Input: part model. Units: mm. Frame: model coordinates. A direction names the side the tool comes from. Give positions to 0.01 mm unless a question says otherwise; leave off trailing zeros. Loops run counter-clockwise (first coordinate to the right, second up) from the corner with the lowest first, then second, coordinate; pieces in that order, holes last. Notation, with made-up numbers: M 50,-1 L 88,-1 A12 cw 88,16 Z; hole C 60,75 d4. An arc over 180 degrees is marked long. One line per item, written item: value. Start each with the question number.
(1) Pin query (flat end, axial travel): P1, Ø0.5, axis at x = 3, z = 10, coming from the -Y side; P2, Ø1.6, axis at x = 40.23, z = 10, coming from the -Y side; P3, Ø4, axis at x = 41, z = 6, coming from the +Y side. Return the tip coordinate at first contact, or that it passes through.
(2) Access query for faces 4 (the flat face through (26.693, 37.246, 9.86)), 5 (the cylindrical face through (39.276, 10.462, 9.7)), 6 (the flat face through (42.53, 10, 10)), 7 (the flat face through (5, 17, 5.5)). Directions: +Z, -Z, +X, -X, +Y, -Y. A direction counts if a zero-diameter tool reaches every point of the face in a straight line with its end or side. Return the directions, or none.
(3) Pull-direction query (Z, two-part tool) for faces 1 (the flat face through (39, 7.997, 10)), 2 (the flat face through (5, 15.843, 10)), 3 (the flat face through (25, 1, 0)); classes: released by +Z, released by -Z, zero draft, split by the parting line, or undercut.
(4) Section D-D on x = 18. Output: boundary loops of the cut face in (y, z).
(5) Section A-A on y = 11. Output: boundary loops of the cut face in (x, z).
(6) Section C-C on x = 27. Output: boundary loops of the cut face in (y, z).
(7) Section B-B on x = 40.23. Output: boundary loops of the cut face in (y, z), plus the area to 3 significant figures.
(8) Ray query, line 1 along X through (y, z) = (11.6, 10); line 2 along Y through (x, z) = (9.5, 6.5); line 3 along Y through (x, z) = (43, 1.5). Return the intervals inside material, ascending. Write a range as from..to.
```python
from build123d import *

# Parameters (mm, degrees)
BOSS_EXTRUDE1_DEPTH = 20
SKETCH5_W           = 9
SKETCH5_H           = 1.454272164
CUT_EXTRUDE4_DEPTH  = 10
SKETCH6_R           = 0.5
CUT_EXTRUDE5_DEPTH  = 5
CUT_EXTRUDE6_DEPTH  = 21
SKETCH11_R          = 1
CUT_EXTRUDE7_DEPTH  = 5


with BuildPart() as part:
    # Sketch1 → Boss-Extrude1 (new body)
    with BuildSketch(Plane.XY):
        with BuildLine():
            Line((0, 29.638125792), (0, -29.638125792))
            ThreePointArc((0, -29.638125792), (3.474436626, -37.215527896), (11.483404529, -39.527489321))
            Line((11.483404529, -39.527489321), (41.483404529, -35.027489321))
            ThreePointArc((41.483404529, -35.027489321), (47.577402104, -31.663689166), (50, -25.138125792))
            Line((50, -25.138125792), (50, 25.138125792))
            ThreePointArc((50, 25.138125792), (47.577402104, 31.663689166), (41.483404529, 35.027489321))
            Line((41.483404529, 35.027489321), (11.483404529, 39.527489321))
            ThreePointArc((11.483404529, 39.527489321), (3.474436626, 37.215527896), (0, 29.638125792))
        make_face()
    extrude(amount=BOSS_EXTRUDE1_DEPTH)

    # Sketch5 → Cut-Extrude4 (cut)
    with BuildSketch(Plane.ZY):
        with Locations((10, 16.569972364)):
            Rectangle(SKETCH5_W, SKETCH5_H)
    extrude(amount=-CUT_EXTRUDE4_DEPTH, mode=Mode.SUBTRACT)

    # Sketch6 → Cut-Extrude5 (cut)
    with BuildSketch(Plane.XZ.offset(-17.297108446)):
        with Locations((2.644871575, 10)):
            Circle(SKETCH6_R)
    extrude(amount=-CUT_EXTRUDE5_DEPTH, mode=Mode.SUBTRACT)

    # Sketch9 → Cut-Extrude6 (cut, through all)
    with BuildSketch(Plane.XY.offset(20)):
        Polygon((42.2, 5.497108446), (42.2, -10.402891554), (50, -10.402891554), (50, 12.297108446), (42.53, 12.297108446), (42.53, 7.997108446), (37.5, 7.997108446), (37.5, 5.497108446), align=None)
    extrude(amount=-CUT_EXTRUDE6_DEPTH, mode=Mode.SUBTRACT)

    # Sketch11 → Cut-Extrude7 (cut)
    with BuildSketch(Plane(origin=(0, 7.997108446, 0), x_dir=(-1, 0, 0), z_dir=(0, -1, 0))):
        with Locations((-40.23, -10)):
            Circle(SKETCH11_R)
    extrude(amount=-CUT_EXTRUDE7_DEPTH, mode=Mode.SUBTRACT)


solid = part.part
```
Output values:
1. P1: stops at y = -37.02
1. P2: stops at y = -35.34
1. P3: stops at y = 35.4
2. face 4: +Z, -Z, +X, +Y
2. face 5: none
2. face 6: +Z, -Z, +X
2. face 7: -X
3. face 1: zero draft
3. face 2: undercut
3. face 3: released by -Z
4. outline: M -38.55,0 L 38.55,0 L 38.55,20 L -38.55,20 Z
5. outline: M 0,0 L 42.53,0 L 42.53,20 L 0,20 Z; hole C 40.23,10 d2
6. outline: M -37.2,0 L 37.2,0 L 37.2,20 L -37.2,20 Z
7. outline: M -35.22,0 L 5.5,0 L 5.5,20 L -35.22,20 Z; M 8,0 L 35.22,0 L 35.22,20 L 8,20 L 8,11 L 13,11 L 13,9 L 8,9 Z
7. area: 1,350 mm²
8. line 1: x = 0..39.23, 41.23..42.53
8. line 2: y = -39.63..15.84, 17.3..39.63
8. line 3: y = -34.68..-10.4, 12.3..34.68
